```python
from build123d import *

# Parameters (mm, degrees)
SKETCH_1_W                   = 80
SKETCH_1_H                   = 50
EXTRUDE_1_DEPTH              = 10
SKETCH_5_R                   = 1.75
CUT_EXTRUDE_1_DEPTH          = 49.218253805
SKETCH_6_R                   = 4
CUT_EXTRUDE_2_DEPTH          = 5
HOLE_WIZARD_M3_1_D           = 3.4
HOLE_WIZARD_M3_1_CSINK_D     = 3.45
HOLE_WIZARD_M3_1_CSINK_ANGLE = 90


with BuildPart() as part:
    # 草图1 → 凸台-拉伸1 (new body)
    with BuildSketch(Plane.XY):
        Rectangle(SKETCH_1_W, SKETCH_1_H)
    extrude(amount=EXTRUDE_1_DEPTH)

    # 草图5 → 切除-拉伸1 (cut, through all)
    with BuildSketch(Plane(origin=(0, 0, 0), x_dir=(-1, 0, 0), z_dir=(0, 0, -1))):
        with Locations((-32, 0)):
            Circle(SKETCH_5_R)
        with Locations((-4, 0)):
            Circle(SKETCH_5_R)
        with Locations((31, 13)):
            Circle(SKETCH_5_R)
        with Locations((31, -19.5)):
            Circle(SKETCH_5_R)
    extrude(amount=-CUT_EXTRUDE_1_DEPTH, mode=Mode.SUBTRACT)

    # 草图6 → 切除-拉伸2 (cut)
    with BuildSketch(Plane.XY.offset(10)):
        with Locations((-31, 13)):
            Circle(SKETCH_6_R)
        with Locations((4, 0)):
            Circle(SKETCH_6_R)
        with Locations((32, 0)):
            Circle(SKETCH_6_R)
        with Locations((-31, -19.5)):
            Circle(SKETCH_6_R)
    extrude(amount=-CUT_EXTRUDE_2_DEPTH, mode=Mode.SUBTRACT)

    # M3 间隙孔1 (through all)
    with Locations(Plane.XY.offset(10)):
        with Locations((-10, 10), (10, 10), (10, -10), (-10, -10)):
            CounterSinkHole(HOLE_WIZARD_M3_1_D / 2, HOLE_WIZARD_M3_1_CSINK_D / 2, counter_sink_angle=HOLE_WIZARD_M3_1_CSINK_ANGLE)


solid = part.part
```
The model under review builds one solid part; all positions refer to its coordinate system, in mm. A direction names the side the tool comes from. Give positions to 0.01 mm unless a question says otherwise; leave off trailing zeros. Write each loop counter-clockwise with the first axis right and the second up, starting at its lowest first coordinate (ties: lowest second). Pieces come first, ordered by that corner, then holes. Notation, with made-up numbers: M -32.75,-38 L -6.75,-38 A30 cw -6.75,-14 Z; hole C 18,-18.5 d6. An arc over 180 degrees is marked long. Write item = value, one per line. Start each with the question number.
Q1. We need section C-C (y = -10). State the section outline as (x, z) points (3 decimals).
Q2. Machinability: for faces 1 (the face through (-29, -20, 5)), 2 (the face through (5.75, 0.08, 2.46)), which of the approach directions +Z, -Z, +X, -X, +Y, -Y give a long, thin tool a straight path to every point of the face, cutting with its end or side? Answer none if there is none.
Q3. We need section D-D (z = 2). Give the number of separate pieces and of enclosed holes in the cut face, plus the area to 3 significant figures.
Q4. Mouldability with a two-part tool opening along Y and no side actions: class faces 3 (the face through (-1, -25, 5)), 4 (the face through (-31.521, 16.966, 7.535)), 5 (the face through (-1, 25, 5)), 6 (the face through (-1, 0, 10)) as released by +Y, released by -Y, zero draft, split by the parting line, or undercut.
Q5. For line 1 (Y direction, x = 10, z = 6.25); line 2 (Y direction, x = -31, z = 1.6); line 3 (Y direction, x = 4, z = 3.9), list the stretches that pass through material, from the lowest coordinate up.
Q6. We need section A-A (x = 32). State the section outline as (y, z) points, plus the area to 4 significant figures.
Q7. We need section B-B (y = 13). State the section outline as (x, z) points, plus the area to 4 significant figures.
Q8. Clearance check with a flat-ended pin moving along its axis: pin 1 (6.5 mm diameter, centred on x = 4, y = 0, fed in from +Z). State where the tip first meets the part, or that it passes through.
Result set:
q1.outline = M -40,0 L -11.7,0 L -11.7,9.975 L -11.725,10 L -40,10 Z; M -8.3,0 L 8.3,0 L 8.3,9.975 L 8.275,10 L -8.275,10 L -8.3,9.975 Z; M 11.7,0 L 40,0 L 40,10 L 11.725,10 L 11.7,9.975 Z
q2.face_1 = +Z
q2.face_2 = +Z, -Z
q3.separate_pieces = 1
q3.enclosed_holes = 8
q3.area = 3,930 mm2
q4.face_3 = released by -Y
q4.face_4 = undercut
q4.face_5 = released by +Y
q4.face_6 = zero draft
q5.line_1 = -25 to -11.7, -8.3 to 8.3, 11.7 to 25
q5.line_2 = -25 to -21.25, -17.75 to 11.25, 14.75 to 25
q5.line_3 = -25 to -1.75, 1.75 to 25
q6.outline = M -25,0 L -1.75,0 L -1.75,5 L -4,5 L -4,10 L -25,10 Z; M 1.75,0 L 25,0 L 25,10 L 4,10 L 4,5 L 1.75,5 Z
q6.area = 442.5 mm2
q7.outline = M -40,0 L -32.75,0 L -32.75,5 L -35,5 L -35,10 L -40,10 Z; M -29.25,0 L 40,0 L 40,10 L -27,10 L -27,5 L -29.25,5 Z
q7.area = 742.5 mm2
q8.pin_1 = 5
